For this review, take the finished solid that the model builds, in its own axes (mm). Coordinates: 2 decimals unless noted, no trailing zeros. Loops run counter-clockwise (first coordinate to the right, second up) from the corner with the lowest first, then second, coordinate; pieces in that order, holes last. Notation, with made-up numbers: (89, 67.25) - (134, 67.25) arc R17 ccw to (134, 87.25) - close; hole circle Ø11 at (13, 65.5). An arc over 180 degrees is marked (long way). Answer as a JSON object with one key per item and string values. Group by question number.
Item 1: We need section C-C (z = 15). Give the boundary of the cut face in (x, y).
Item 2: We need section B-B (x = 19). Give the boundary of the cut face in (y, z).
Item 3: We need section A-A (z = 63.5). Give the boundary of the cut face in (x, y).
Item 4: We need section D-D (y = 2.4). State how many separate pieces and enclosed holes the cut face has, then the cut area to 3 significant figures.
Item 5: Clearance check with flat-ended pins moving along their axes: pin 1 (1.5 mm diameter, centred on y = 1, z = 73.5, fed in from +X); pin 2 (0.9 mm diameter, centred on y = 1, z = -72.5, fed in from -X); pin 3 (1.6 mm diameter, centred on x = -69, y = 1.5, fed in from -Z); pin 4 (2.5 mm diameter, centred on x = 95.5, z = -69.5, fed in from +Y). State where each tip first meets the part, or that it passes through.
Item 6: To check wall thickness, follow line 1 (X direction, y = 1.2, z = -20.5); line 2 (X direction, y = 0.6, z = 19.9); line 3 (Z direction, x = 89.92, y = 2.2). State the ranges of each line that lie inside material, in increasing order.
from build123d import *

# Parameters (mm, degrees)
SKETCH1_W           = 200
SKETCH1_H           = 151
BOSS_EXTRUDE1_DEPTH = 3
SKETCH2_W           = 28.1297743
SKETCH2_H           = 36.772110208
SKETCH2_R           = 1.5
SKETCH2_R_2         = 1.4
CUT_EXTRUDE2_DEPTH  = 4
FILLET1_R           = 5


with BuildPart() as part:
    # Sketch1 → Boss-Extrude1 (new body)
    with BuildSketch(Plane(origin=(0, 0, 0), x_dir=(1, 0, 0), z_dir=(0, 1, 0))):
        Rectangle(SKETCH1_W, SKETCH1_H)
    extrude(amount=BOSS_EXTRUDE1_DEPTH)

    # Sketch2 → Cut-Extrude2 (cut, through all)
    with BuildSketch(Plane(origin=(0, 3, 0), x_dir=(1, 0, 0), z_dir=(0, 1, 0))):
        Polygon((-50, 75.5), (-81, 75.5), (-81, 71), (-68, 71), (-68, 58.75), (-69.5, 58.75), (-69.5, 55.25), (-68, 55.25), (-68, 47.5), (-63, 47.5), (-63, 55.25), (-61.5, 55.25), (-61.5, 58.75), (-63, 58.75), (-63, 71), (-50, 71), align=None)
        Polygon((50, 71), (63, 71), (63, 58.75), (61.5, 58.75), (61.5, 55.25), (63, 55.25), (63, 47.5), (68, 47.5), (68, 55.25), (69.5, 55.25), (69.5, 58.75), (68, 58.75), (68, 71), (81, 71), (81, 75.5), (50, 75.5), align=None)
        Polygon((50, -75.5), (81, -75.5), (81, -71), (68, -71), (68, -58.75), (69.5, -58.75), (69.5, -55.25), (68, -55.25), (68, -47.5), (63, -47.5), (63, -55.25), (61.5, -55.25), (61.5, -58.75), (63, -58.75), (63, -71), (50, -71), align=None)
        Polygon((-50, -71), (-63, -71), (-63, -58.75), (-61.5, -58.75), (-61.5, -55.25), (-63, -55.25), (-63, -47.5), (-68, -47.5), (-68, -55.25), (-69.5, -55.25), (-69.5, -58.75), (-68, -58.75), (-68, -71), (-81, -71), (-81, -75.5), (-50, -75.5), align=None)
        with Locations((19.572588651, -8.701882989)):
            Rectangle(SKETCH2_W, SKETCH2_H)
        with Locations((89.92, -19.9)):
            Circle(SKETCH2_R)
        with Locations((89.92, 11.61)):
            Circle(SKETCH2_R)
        with Locations((58.16, 4)):
            Circle(SKETCH2_R)
        with Locations((95.5, 20.5)):
            Circle(SKETCH2_R_2)
        with Locations((37.5, 20.5)):
            Circle(SKETCH2_R_2)
        with Locations((37.5, 69.5)):
            Circle(SKETCH2_R_2)
        with Locations((95.5, 69.5)):
            Circle(SKETCH2_R_2)
    extrude(amount=-CUT_EXTRUDE2_DEPTH, mode=Mode.SUBTRACT)

    # Fillet1
    fillet1_edges = [part.edges().sort_by_distance(p)[0] for p in [
        (100, 1.5, 75.5),
        (-100, 1.5, 75.5),
        (-100, 1.5, -75.5),
        (100, 1.5, -75.5),
    ]]
    fillet(fillet1_edges, radius=FILLET1_R)


solid = part.part
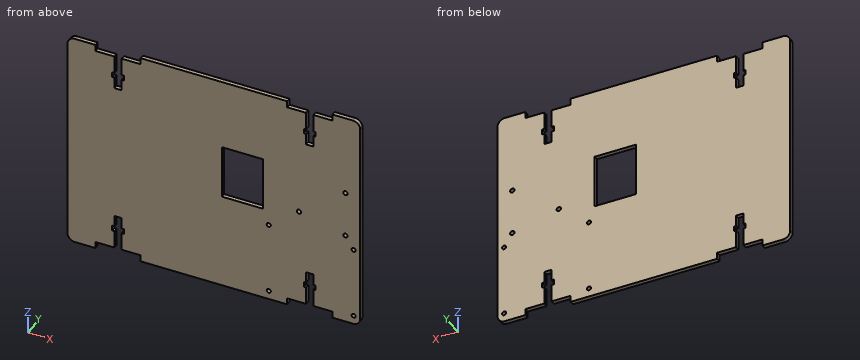
Check sheet entries:
{
 "1": {"outline": "(-100, 0) - (5.51, 0) - (5.51, 3) - (-100, 3) - close; (33.64, 0) - (100, 0) - (100, 3) - (33.64, 3) - close"},
 "2": {"outline": "(0, -75.5) - (3, -75.5) - (3, -9.68) - (0, -9.68) - close; (0, 27.09) - (3, 27.09) - (3, 75.5) - (0, 75.5) - close"},
 "3": {"outline": "(-100, 0) - (-68, 0) - (-68, 3) - (-100, 3) - close; (-63, 0) - (63, 0) - (63, 3) - (-63, 3) - close; (68, 0) - (100, 0) - (100, 3) - (68, 3) - close"},
 "4": {"separate pieces": "1", "enclosed holes": "8", "area": "28,000 mm2"},
 "5": {"pin 1": "stops at x = 99.47", "pin 2": "stops at x = -99.75", "pin 3": "stops at z = -71", "pin 4": "passes through"},
 "6": {"line 1": "x = -100 to 36.1, 38.9 to 94.1, 96.9 to 100", "line 2": "x = -100 to 5.51, 33.64 to 88.42, 91.42 to 100", "line 3": "z = -75.5 to -13.11, -10.11 to 18.4, 21.4 to 75.5"}
}
